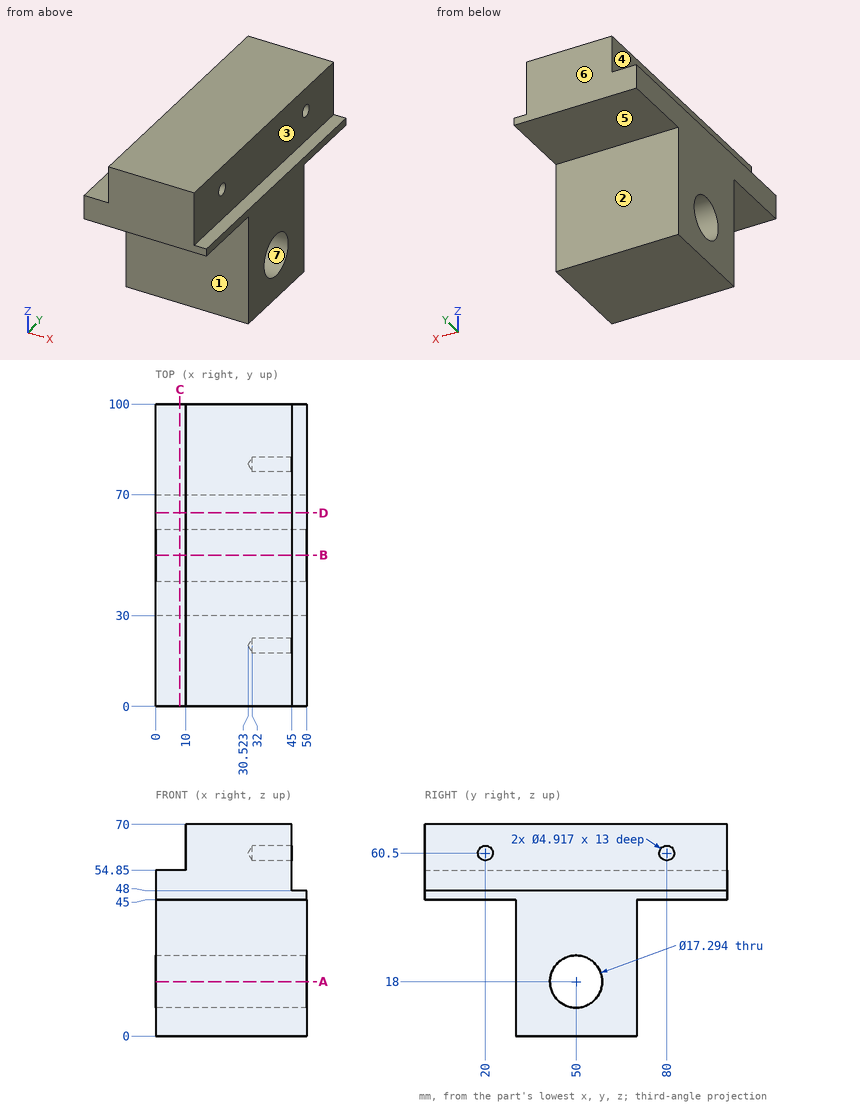
The drawing under review shows one solid part. Ordinate dimensions are in mm from its lowest x, y, z. A direction names the side the tool comes from. Give positions to 0.01 mm unless a question says otherwise; leave off trailing zeros. Write each loop counter-clockwise with the first axis right and the second up, starting at its lowest first coordinate (ties: lowest second). Pieces come first, ordered by that corner, then holes. Notation, with made-up numbers: (57, -14.5) -> (111, -14.5) arc R21 cw to (111, 6.5) -> close; hole circle Ø9 at (47.25, -26). An arc over 180 degrees is marked (long way). Put each result on its own line as item: value.
(1) We need section A-A, the plane z = 18. Give the boundary of the cut face in (x, y), and give its area (3 significant figures).
Results are:
outline: (0, 30) -> (50, 30) -> (50, 41.35) -> (0, 41.35) -> close; (0, 58.65) -> (50, 58.65) -> (50, 70) -> (0, 70) -> close
area: 1,140 mm²
(2) We need section D-D, the plane y = 64. Give the boundary of the cut face in (x, z).
Results are:
outline: (0, 0) -> (50, 0) -> (50, 48) -> (45, 48) -> (45, 70) -> (10, 70) -> (10, 54.85) -> (0, 54.85) -> close
(3) To check wall thickness, follow probe 1 along Y at (x, z) = (35, 60.5); probe 2 along Z at (x, y) = (12, 50); probe 3 along Z at (x, y) = (36, 20). State the ranges of each line that lie inside material, in increasing order. Write a range as from..to.
Results are:
probe 1: 0..17.54, 22.46..77.54, 82.46..100
probe 2: 0..9.35, 26.65..70
probe 3: 45..58.04, 62.96..70
(4) Tool access review of the marked faces 1, 2, 3 and 4: name each direction out of +Z, -Z, +X, -X, +Y, -Y from which nothing blocks a thin tool from reaching the whole face with its end or side.
Results are:
face 1: -Z, +X, -X, -Y
face 2: -Z, +X, -X, +Y
face 3: +Z, +X, +Y, -Y
face 4: +Z, -X, +Y, -Y
(5) The part is to be moulded in two halves that separate along Y. For the marked faces 5, 6 and 7, say which applies: pulls with the +Y half, pulls with the -Y half, needs draft (parallel to the pull), parting line crosses it, or undercut.
Results are:
face 5: needs draft
face 6: pulls with the +Y half
face 7: undercut
(6) We need section B-B, the plane y = 50. Give the boundary of the cut face in (x, z), and give its area (3 significant figures).
Results are:
outline: (0, 0) -> (50, 0) -> (50, 9.35) -> (0, 9.35) -> close; (0, 26.65) -> (50, 26.65) -> (50, 48) -> (45, 48) -> (45, 70) -> (10, 70) -> (10, 54.85) -> (0, 54.85) -> close
area: 2,370 mm²
(7) For pin 1 Ø12 at (x, z) = (38.5, 34) entering from -Y; pin 2 Ø12 at (y, z) = (38, 64.5) entering from -X; pin 3 Ø4.5 at (y, z) = (20, 60.5) entering from +X (1 decimal), all flat-tipped, find the tip position at first contact; note any pin that passes through.
Results are:
pin 1: y = 30
pin 2: x = 10
pin 3: x = 31.9
(8) We need section C-C, the plane x = 8. Give the boundary of the cut face in (y, z).
Results are:
outline: (0, 45) -> (30, 45) -> (30, 0) -> (70, 0) -> (70, 45) -> (100, 45) -> (100, 54.85) -> (0, 54.85) -> close; hole circle Ø17.29 at (50, 18)
